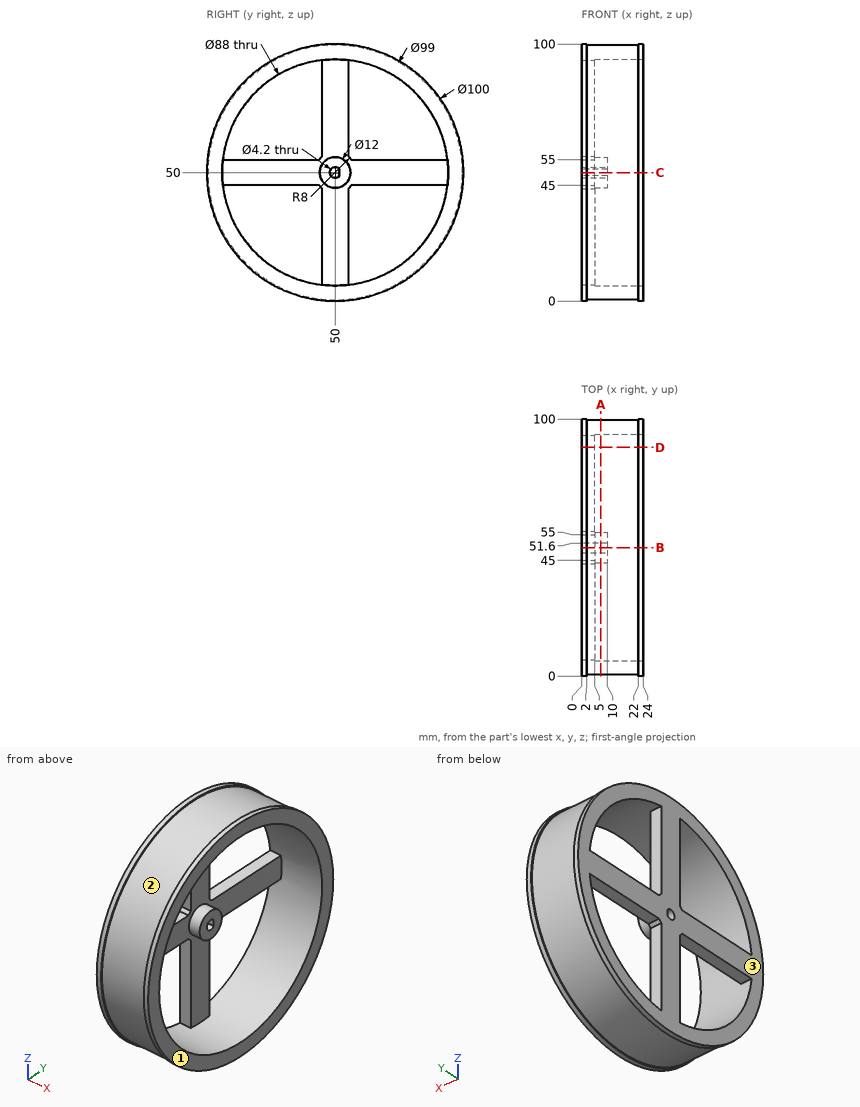
Design review of the part shown in the three views and the two pictorial views. Dimensions are in mm from the part's minimum x, y and z. Coordinates: 2 decimals unless noted, no trailing zeros. Loops run counter-clockwise (first coordinate to the right, second up) from the corner with the lowest first, then second, coordinate; pieces in that order, holes last.
(1) Consider section B-B, the plane y = 50. Give the boundary of the cut face in (x, z).
Determined:
outline: (0, 0) - (2, 0) - (2, 0.5) - (22, 0.5) - (22, 0) - (24, 0) - (24, 6) - (5, 6) - (5, 44) - (10, 44) - (10, 47.9) - (0, 47.9) - close; (0, 52.1) - (10, 52.1) - (10, 56) - (5, 56) - (5, 94) - (24, 94) - (24, 100) - (22, 100) - (22, 99.5) - (2, 99.5) - (2, 100) - (0, 100) - close
(2) Insertion check: P1, Ø4, axis at x = 3, y = 69, coming from the -Z side; P2, Ø2.5, axis at x = 2, z = 22, coming from the +Y side; P3, Ø4, axis at y = 50, z = 50, coming from the +X side. Each pin has a flat end and moves straight along its axis. Give the tip position at first contact, or say it passes through.
Determined:
P1: stops at z = 3.08
P2: stops at y = 92.24
P3: stops at x = 10
(3) Draft analysis for pull direction X (two halves, no side actions). For the marked faces 1, 2 and 3, state which applies: +X half, -X half, draft (parallel to the pull), parting line (faces both ways), or undercut.
Determined:
face 1: +X half
face 2: undercut
face 3: -X half
(4) Consider section C-C, the plane z = 50. Give the boundary of the cut face in (x, y).
Determined:
outline: (0, 0) - (2, 0) - (2, 0.5) - (22, 0.5) - (22, 0) - (24, 0) - (24, 6) - (5, 6) - (5, 44) - (10, 44) - (10, 47.9) - (0, 47.9) - close; (0, 51.6) - (10, 51.6) - (10, 56) - (5, 56) - (5, 94) - (24, 94) - (24, 100) - (22, 100) - (22, 99.5) - (2, 99.5) - (2, 100) - (0, 100) - close
(5) Consider section A-A, the plane x = 7.5. Give the boundary of the cut face in (y, z).
Determined:
outline: circle Ø99 at (50, 50); circle Ø12 at (50, 50); hole circle Ø88 at (50, 50); hole (51.6, 48.64) - (51.6, 51.36) arc R2.1 ccw (long way) to start
(6) Consider section D-D, the plane y = 89. Give the boundary of the cut face in (x, z).
Determined:
outline: (0, 18.71) - (2, 18.71) - (2, 19.52) - (22, 19.52) - (22, 18.71) - (24, 18.71) - (24, 29.63) - (0, 29.63) - close; (0, 45) - (5, 45) - (5, 55) - (0, 55) - close; (0, 70.37) - (24, 70.37) - (24, 81.29) - (22, 81.29) - (22, 80.48) - (2, 80.48) - (2, 81.29) - (0, 81.29) - close
(7) Wall thickness on L1, parallel to Z at x = 6.5, y = 50; L2, parallel to Y at x = 6.25, z = 54.5; L3, parallel to Z at x = 2.75, y = 50: over which ranges is each line inside the solid? List them lowest first.
Determined:
L1: z = 0.5 to 6, 44 to 47.9, 52.1 to 56, 94 to 99.5
L2: y = 0.7 to 6.23, 46.03 to 53.97, 93.77 to 99.3
L3: z = 0.5 to 47.9, 52.1 to 99.5
